Answer from the drawing. Dimensions are ordinates in mm from the lowest x, y and z of the part. A direction names the side the tool comes from. Give positions to 0.01 mm unless a question says otherwise; leave off trailing zeros. Loops run counter-clockwise (first coordinate to the right, second up) from the corner with the lowest first, then second, coordinate; pieces in that order, holes last. Notation, with made-up numbers: M 29,19 L 62,19 A9 ccw 62,23 Z; hole C 21,46.5 d5. An arc over 180 degrees is marked long. Return JSON: item names as keys, results as strings. Group by question number.
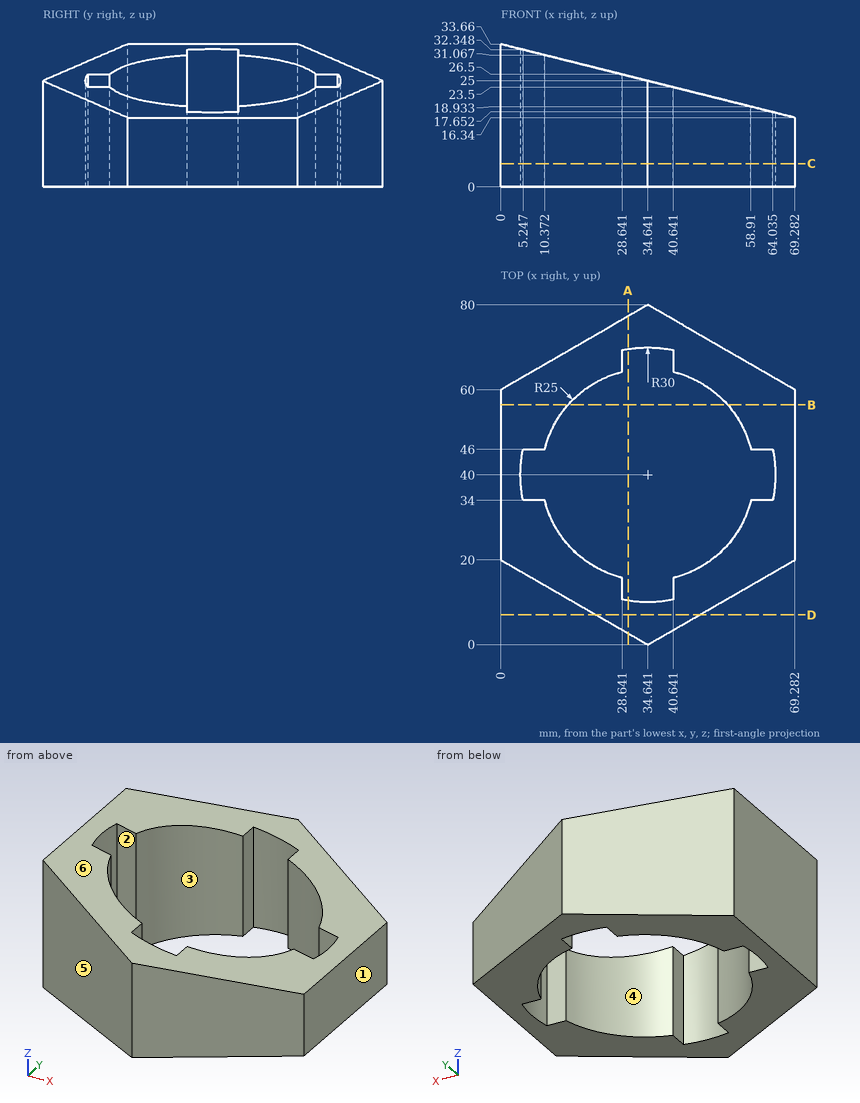
1. Find section C-C (z = 5.5). Write down the section's boundary in (x, y) (1 decimal), and give its area (3 significant figures).
2. The mould has two halves that part along Y. Classify the marked faces 3, 4, 5 and 6: +Y half, -Y half, draft (parallel to the pull), parting line (faces both ways), or undercut.
3. For the marked faces 1 and 2, determine the directions among +Z, -Z, +X, -X, +Y, -Y from which every point of the face is accessible in a straight line to the end or side of a thin tool.
4. Straight lines are drawn through the part: line 1 along Y through (x, z) = (8, 9.5); line 2 along Y through (x, z) = (17.5, 29) (1 decimal); line 3 along Z through (x, y) = (20, 9.5). For each, find the intervals that lie inside material, in ascending order.
5. Flat-ended cylindrical pins translate along their axes: P1, Ø4, axis at x = 6.5, z = 8.5, coming from the +Y side; P2, Ø1.5, axis at y = 27, z = 24.5, coming from the +X side; P3, Ø5.5, axis at x = 60.5, z = 9.5, coming from the -Y side. Find the tip coordinate at first contact, or state that the pin passes through.
6. Find section B-B (y = 56.5). Write down the section's boundary in (x, z) (1 decimal), and give its area (3 significant figures).
7. Find section A-A (x = 30). Write down the section's boundary in (y, z).
8. Find section D-D (y = 7). Write down the section's boundary in (x, z) (1 decimal), and give its area (3 significant figures).
Result:
{
 "1": {"outline": "M 0,20 L 34.6,0 L 69.3,20 L 69.3,60 L 34.6,80 L 0,60 Z; hole M 5.2,34 L 10.4,34 A25 ccw 28.6,15.7 L 28.6,10.6 A30 ccw 40.6,10.6 L 40.6,15.7 A25 ccw 58.9,34 L 64,34 A30 ccw 64,46 L 58.9,46 A25 ccw 40.6,64.3 L 40.6,69.4 A30 ccw 28.6,69.4 L 28.6,64.3 A25 ccw 10.4,46 L 5.2,46 A30 ccw Z", "area": "1,950 mm2"},
 "2": {"face 3": "undercut", "face 4": "undercut", "face 5": "-Y half", "face 6": "draft"},
 "3": {"face 1": "+Z, -Z, +X, +Y, -Y", "face 2": "+Z, -Z"},
 "4": {"line 1": "y = 15.38 to 34, 46 to 64.62", "line 2": "y = 9.9 to 21.8, 58.2 to 70.1", "line 3": "z = 0 to 28.66"},
 "5": {"P1": "stops at y = 64.91", "P2": "stops at x = 13.76", "P3": "stops at y = 13.34"},
 "6": {"outline": "M 0,0 L 15.9,0 L 15.9,29.7 L 0,33.7 Z; M 53.4,0 L 69.3,0 L 69.3,16.3 L 53.4,20.3 Z", "area": "793 mm2"},
 "7": {"outline": "M 2.68,0 L 10.36,0 L 10.36,26.16 L 2.68,26.16 Z; M 69.64,0 L 77.32,0 L 77.32,26.16 L 69.64,26.16 Z"},
 "8": {"outline": "M 22.5,0 L 46.8,0 L 46.8,22 L 22.5,28 Z", "area": "606 mm2"}
}
